Part model, mm, in its own coordinate system. Face numbers are marked on the shaded views. A direction names the side the tool comes from. Round coordinates to 2 decimals unless told otherwise and drop trailing zeros. Write each loop counter-clockwise with the first axis right and the second up, starting at its lowest first coordinate (ties: lowest second). Pieces come first, ordered by that corner, then holes. Notation, with made-up numbers: (-23, 23.25) -> (32, 23.25) arc R25 cw to (32, 60.25) -> close; hole circle Ø9 at (3, -24.75). An arc over 180 degrees is marked (long way). Return JSON: item names as keys, results as strings. Group by question number.
(1) Saw through at D-D (y = 7.75). List the corners of the cut face in (x, z).
(2) Saw through at A-A (y = 24.75). List the corners of the cut face in (x, z), plus the area to 3 significant figures.
(3) Saw through at C-C (z = -1). List the corners of the cut face in (x, y).
(4) Drop flat-ended pins along their axis: pin 1 Ø17 at (x, z) = (-20.5, -1.5) entering from -Y; pin 2 Ø11 at (x, y) = (-16, 20.5) entering from +Z; pin 3 Ø5 at (y, z) = (7, -1.5) entering from -X; pin 4 Ø8 at (x, z) = (-13.5, 18) entering from -Y. Give the stop position or say it passes through.
(5) Saw through at B-B (x = 29). List the corners of the cut face in (y, z).
(6) Drill centre lines: L1, parallel to Y at x = -11, z = 9; L2, parallel to X at y = 3.75, z = 10.5; L3, parallel to Y at x = 5, z = -20.5. Where is each one in solid material? Low to high. Write a range as from..to.
(7) Mould opens along Z. For the marked faces 6, 7, 8 and 9 say: +Z half, -Z half, draft (parallel to the pull), parting line (faces both ways), or undercut.
(8) Tool access for the marked faces 1, 2, 3, 4 and 5: list every direction of +Z, -Z, +X, -X, +Y, -Y with a clear straight run to the whole face (end or side of a thin tool).
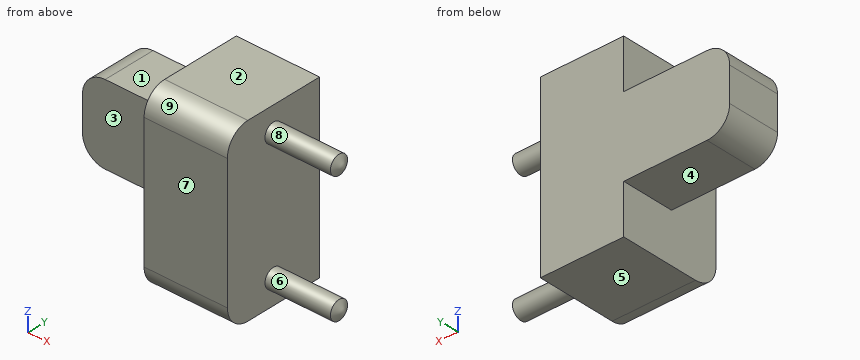
from build123d import *

# Parameters (mm, degrees)
SKIZZE1_W                       = 22
SKIZZE1_H                       = 47.002
AUFSATZ_LINEAR_AUSTRAGEN1_DEPTH = 27
VERRUNDUNG1_R                   = 6
SKIZZE2_W                       = 21
SKIZZE2_H                       = 14
AUFSATZ_LINEAR_AUSTRAGEN2_DEPTH = 28
VERRUNDUNG2_R                   = 6
SKIZZE3_R                       = 2.5
AUFSATZ_LINEAR_AUSTRAGEN3_DEPTH = 17.3


with BuildPart() as part:
    # Skizze1 → Aufsatz-Linear austragen1 (new body)
    with BuildSketch(Plane(origin=(0, 0, 0), x_dir=(1, 0, 0), z_dir=(0, 1, 0))):
        with Locations((11, 0)):
            Rectangle(SKIZZE1_W, SKIZZE1_H)
    extrude(amount=AUFSATZ_LINEAR_AUSTRAGEN1_DEPTH)

    # Verrundung1
    verrundung1_edges = [part.edges().sort_by_distance(p)[0] for p in [
        (11, 0, -23.501),
        (11, 0, 23.501),
    ]]
    fillet(verrundung1_edges, radius=VERRUNDUNG1_R)

    # Skizze2 → Aufsatz-Linear austragen2 (add)
    with BuildSketch(Plane.ZY):
        with Locations((0, 20)):
            Rectangle(SKIZZE2_W, SKIZZE2_H)
    extrude(amount=AUFSATZ_LINEAR_AUSTRAGEN2_DEPTH)

    # Verrundung2
    verrundung2_edges = [part.edges().sort_by_distance(p)[0] for p in [
        (-28, 20, -10.5),
        (-28, 20, 10.5),
    ]]
    fillet(verrundung2_edges, radius=VERRUNDUNG2_R)

    # Skizze3 → Aufsatz-Linear austragen3 (add)
    with BuildSketch(Plane(origin=(22, 0, 0), x_dir=(0, 0, -1), z_dir=(1, 0, 0))):
        with Locations(Location((17, 13.5, 0), (0, 0, 180))):
            Circle(SKIZZE3_R)
        with Locations(Location((-17, 13.5, 0), (0, 0, 180))):
            Circle(SKIZZE3_R)
    extrude(amount=AUFSATZ_LINEAR_AUSTRAGEN3_DEPTH)

    # Skizze4 → Rotation2 (revolve)
    with BuildSketch(Plane(origin=(0, 13.5, 0), x_dir=(-1, 0, 0), z_dir=(0, 1, 0)), mode=Mode.PRIVATE) as rotation2_sk:
        Polygon((-39.3, 14.5), (-40.802151548, 17), (-39.3, 17), align=None)
    revolve(rotation2_sk.sketch.rotate(Axis((39.3, 13.5, 17), (1, 0, 0)), 180), axis=Axis((39.3, 13.5, 17), (1, 0, 0)))

    # Skizze5 → Rotation3 (revolve)
    with BuildSketch(Plane(origin=(0, 13.5, 0), x_dir=(-1, 0, 0), z_dir=(0, 1, 0)), mode=Mode.PRIVATE) as rotation3_sk:
        Polygon((-39.3, -19.5), (-39.3, -17), (-40.802151548, -17), align=None)
    revolve(rotation3_sk.sketch.rotate(Axis((39.3, 13.5, -17), (1, 0, 0)), 180), axis=Axis((39.3, 13.5, -17), (1, 0, 0)))


solid = part.part
Computed values:
{
 "1": {"outline": "(0, -23.5) -> (22, -23.5) -> (22, 23.5) -> (0, 23.5) -> close"},
 "2": {"outline": "(-28, -4.5) arc R6 ccw to (-22, -10.5) -> (0, -10.5) -> (0, -23.5) -> (22, -23.5) -> (22, 23.5) -> (0, 23.5) -> (0, 10.5) -> (-22, 10.5) arc R6 ccw to (-28, 4.5) -> close", "area": "1,610 mm2"},
 "3": {"outline": "(-28, 13) -> (0, 13) -> (0, 0) -> (22, 0) -> (22, 27) -> (-28, 27) -> close"},
 "4": {"pin 1": "y = 13", "pin 2": "z = 10.5", "pin 3": "x = 0", "pin 4": "through"},
 "5": {"outline": "circle Ø5 at (13.5, -17); circle Ø5 at (13.5, 17)"},
 "6": {"L1": "13..27", "L2": "0..22", "L3": "0.8..27"},
 "7": {"face 6": "undercut", "face 7": "draft", "face 8": "undercut", "face 9": "+Z half"},
 "8": {"face 1": "+Z, -X, +Y, -Y", "face 2": "+Z, +X, -X, +Y, -Y", "face 3": "+Z, -Z, -X, -Y", "face 4": "-Z, -X, +Y, -Y", "face 5": "-Z, +X, -X, +Y, -Y"}
}
